Could you check a few things on this model? Use its own coordinates, in mm. Face numbers are marked on the shaded views. Give positions to 0.01 mm unless a question says otherwise; leave off trailing zeros. Order: outer loops, then holes, each group sorted by start corner. A loop starts at its lowest first (then second) coordinate and runs counter-clockwise, first axis right, second up. Notation, with made-up numbers: M -7.75,71.25 L 29.25,71.25 A21 ccw 29.25,102.25 Z; hole C -7,-29 d7. An arc over 180 degrees is marked long. Use a Markdown table: item, result. Add a question column.
Item 1: If I drill on L1, parallel to Z at x = 3.5, y = 10; L2, parallel to Z at x = 5, y = 11.75; L3, parallel to X at y = 9.5, z = -6.5 (3 decimals), over which ranges is the centre line in solid material (lowest first)? Write a range as from..to.
Item 2: Suppose I cut it at B-B on y = 7. Count the separate pieces of the cut face and the enclosed holes in it, plus the area to 3 significant figures.
Item 3: Suppose I cut it at C-C on x = -9. Write out the boundary of the cut face in (y, z).
Item 4: I'm going to push a flat-ended pin straight in: pin 1 Ø2 at (x, z) = (3.48, -6.35) entering from -Y. Where does the tip first touch, or does it pass through?
Item 5: If we mould it in two halves opening along X, with no side actions, what happens to the marked faces 1, 2, 3 and 4? For each: released by +X, released by -X, zero draft, split by the parting line, or undercut.
Item 6: Suppose I cut it at A-A on z = 6.35. Write out the boundary of the cut face in (x, y) (3 decimals).
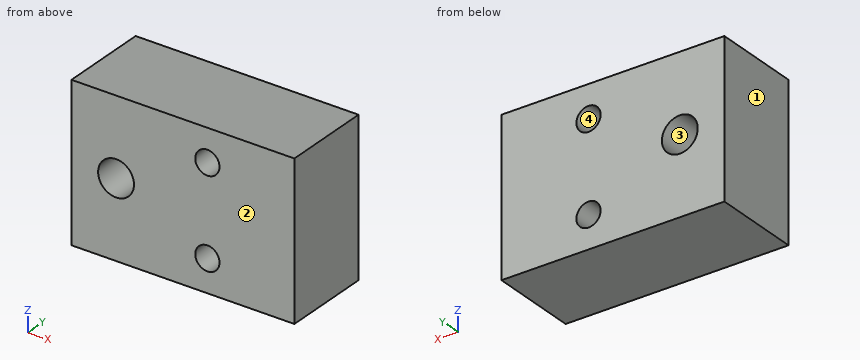
from build123d import *

# Parameters (mm, degrees)
F0_W     = 3.4798
F0_H     = 6.35
F0_W_2   = 12.3952
F1_DEPTH = 12.7
F2_D     = 3.4544
F4_D     = 5.1054


# Not quite as in the source:
# - a feature names something its author has since deleted; it is built from what else it names


with BuildPart() as f1:
    # F0 (on Front) → F1 (new body)
    with BuildSketch(Plane.XZ):
        Polygon((0, -6.35), (0, 0), (-15.875, 0), (-15.875, -10.9855), (0, -10.9855), align=None)
        Polygon((-15.875, 0), (0, 0), (0, 6.35), (0, 10.9855), (-15.875, 10.9855), align=None)
        Polygon((0, 10.9855), (0, 6.35), (3.4798, 6.35), (15.875, 6.35), (15.875, 10.9855), align=None)
        with Locations((1.7399, 3.175)):
            Rectangle(F0_W, F0_H)
        with Locations((9.6774, 3.175)):
            Rectangle(F0_W_2, F0_H)
        with Locations((9.6774, -3.175)):
            Rectangle(F0_W_2, F0_H)
        with Locations((1.7399, -3.175)):
            Rectangle(F0_W, F0_H)
        Polygon((3.4798, -6.35), (0, -6.35), (0, -10.9855), (15.875, -10.9855), (15.875, -6.35), align=None)
    extrude(amount=-F1_DEPTH)

    # F2 (through all)
    with Locations(Plane.XZ):
        with Locations((3.4798, -6.35), (3.4798, 6.35)):
            Hole(F2_D / 2)

    # F4 (through all)
    with Locations(Plane(origin=(0, 12.7, 0), x_dir=(-1, 0, 0), z_dir=(0, 1, 0))):
        with Locations((9.525, 0)):
            Hole(F4_D / 2)


solid = f1.part
Findings below:
| question | item | result |
|---|---|---|
| 1 | L1 | z = -10.99..-8.08, -4.62..4.62, 8.08..10.99 |
| 1 | L2 | z = -10.99..-7.17, -5.53..5.53, 7.17..10.99 |
| 1 | L3 | x = -15.875..1.759, 5.2..15.875 |
| 2 | separate pieces | 1 |
| 2 | enclosed holes | 3 |
| 2 | area | 658 mm^2 |
| 3 | outline | M 0,-10.99 L 12.7,-10.99 L 12.7,-2.5 L 0,-2.5 Z; M 0,2.5 L 12.7,2.5 L 12.7,10.99 L 0,10.99 Z |
| 4 | pin 1 | passes through |
| 5 | face 1 | released by -X |
| 5 | face 2 | zero draft |
| 5 | face 3 | undercut |
| 5 | face 4 | undercut |
| 6 | outline | M -15.875,0 L 1.753,0 L 1.753,12.7 L -15.875,12.7 Z; M 5.207,0 L 15.875,0 L 15.875,12.7 L 5.207,12.7 Z |
